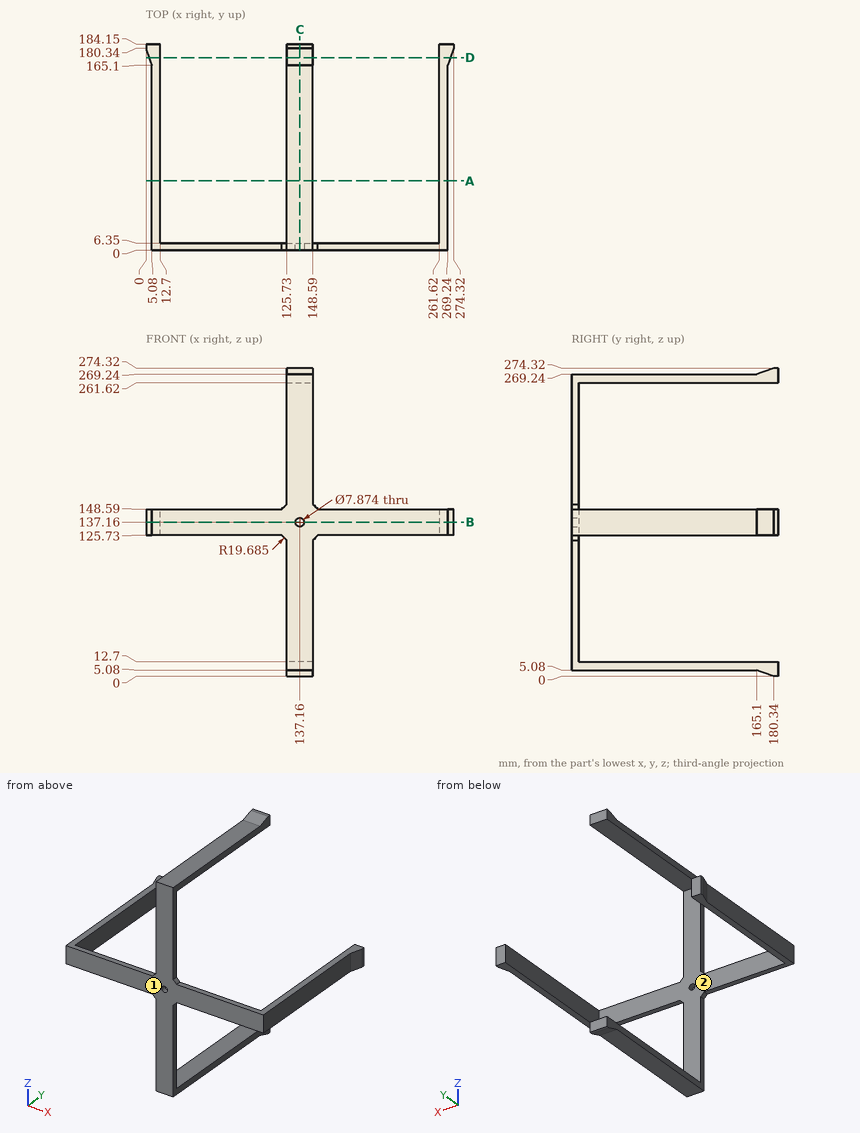
Can you work these out from the drawing? Everything is in mm from the part's minimum corner. Round coordinates to 2 decimals unless told otherwise and drop trailing zeros. Write each loop counter-clockwise with the first axis right and the second up, starting at its lowest first coordinate (ties: lowest second). Pieces come first, ordered by that corner, then holes. Notation, with made-up numbers: (-8, -20.5) - (38, -20.5) arc R21 ccw to (38, 7.5) - close; hole circle Ø8 at (10.5, 23.5). An arc over 180 degrees is marked (long way). Put each result on its own line as item: value. Start each with the question number.
(1) Will these pins go through, and if not, where does the flat tip stop? pin 1 (7 mm diameter, centred on y = 100.5, z = 138, fed in from -X); pin 2 (10 mm diameter, centred on x = 137.16, z = 137.16, fed in from +Y); pin 3 (2 mm diameter, centred on x = 75, z = 126, fed in from -Y); pin 4 (25 mm diameter, centred on x = 141.5, y = 112.5, fed in from -Z).
(2) Thinking about a two-plate mould opening in X: for the marked faces 1 and 2, which applies, released by +X, released by -X, zero draft, split by the parting line, or undercut?
(3) I want a section at D-D, the plane y = 172. Please give me the cut outline in (x, z).
(4) I want a section at A-A, the plane y = 62. Please give me the cut outline in (x, z), plus the area to 3 significant figures.
(5) I want a section at B-B, the plane z = 137.16. Please give me the cut outline in (x, y).
(6) I want a section at C-C, the plane x = 137.16. Please give me the cut outline in (y, z), plus the area to 3 significant figures.
(7) I need wall thicknesses on probe 1 along X at (y, z) = (137, 143.5); probe 2 along X at (y, z) = (4.5, 137.16). Which ranges of each line are inside material? Lowest first, please.
Here are the results:
1. pin 1: stops at x = 5.08
1. pin 2: stops at y = 6.35
1. pin 3: stops at y = 0
1. pin 4: stops at z = 5.08
2. face 1: zero draft
2. face 2: undercut
3. outline: (2.78, 125.73) - (12.7, 125.73) - (12.7, 148.59) - (2.78, 148.59) - close; (125.73, 2.78) - (148.59, 2.78) - (148.59, 12.7) - (125.73, 12.7) - close; (125.73, 261.62) - (148.59, 261.62) - (148.59, 271.54) - (125.73, 271.54) - close; (261.62, 125.73) - (271.54, 125.73) - (271.54, 148.59) - (261.62, 148.59) - close
4. outline: (5.08, 125.73) - (12.7, 125.73) - (12.7, 148.59) - (5.08, 148.59) - close; (125.73, 5.08) - (148.59, 5.08) - (148.59, 12.7) - (125.73, 12.7) - close; (125.73, 261.62) - (148.59, 261.62) - (148.59, 269.24) - (125.73, 269.24) - close; (261.62, 125.73) - (269.24, 125.73) - (269.24, 148.59) - (261.62, 148.59) - close
4. area: 697 mm^2
5. outline: (0, 180.34) - (5.08, 165.1) - (5.08, 0) - (133.22, 0) - (133.22, 6.35) - (12.7, 6.35) - (12.7, 184.15) - (0, 184.15) - close; (141.1, 0) - (269.24, 0) - (269.24, 165.1) - (274.32, 180.34) - (274.32, 184.15) - (261.62, 184.15) - (261.62, 6.35) - (141.1, 6.35) - close
6. outline: (0, 5.08) - (165.1, 5.08) - (180.34, 0) - (184.15, 0) - (184.15, 12.7) - (6.35, 12.7) - (6.35, 133.22) - (0, 133.22) - close; (0, 141.1) - (6.35, 141.1) - (6.35, 261.62) - (184.15, 261.62) - (184.15, 274.32) - (180.34, 274.32) - (165.1, 269.24) - (0, 269.24) - close
6. area: 4,450 mm^2
7. probe 1: x = 5.08 to 12.7, 261.62 to 269.24
7. probe 2: x = 5.08 to 133.22, 141.1 to 269.24
